Work out the finished part from the listing and answer in its coordinate system (mm). A direction names the side the tool comes from. Coordinates: 2 decimals unless noted, no trailing zeros. Order: outer loops, then holes, each group sorted by start corner. A loop starts at its lowest first (then second) coordinate and runs counter-clockwise, first axis right, second up. Notation, with made-up numbers: M -18.5,76.5 L -7.5,76.5 A6 ccw -7.5,81.5 Z; hole C 41,13 d10. An arc over 180 degrees is marked long. Use a Markdown table: item, result. Add a question column.
from build123d import *

# Parameters (mm, degrees)
SKETCH1_W           = 25
SKETCH1_H           = 25
BOSS_EXTRUDE1_DEPTH = 25
SHELL1_T            = 2.5
SKETCH2_W           = 12
SKETCH2_H           = 12
CUT_EXTRUDE1_DEPTH  = 15
SKETCH3_R           = 1.75
CUT_EXTRUDE2_DEPTH  = 15
SKETCH4_R           = 2.5
CUT_EXTRUDE6_DEPTH  = 15
SKETCH4_3_R         = 2.5
CUT_EXTRUDE7_DEPTH  = 15
SKETCH5_R           = 2.5
CUT_EXTRUDE8_DEPTH  = 15
SKETCH5_4_R         = 2.5
CUT_EXTRUDE9_DEPTH  = 15
SKETCH5_5_R         = 2.5
CUT_EXTRUDE10_DEPTH = 15
SKETCH7_R           = 2.5
CUT_EXTRUDE11_DEPTH = 15
SKETCH8_R           = 2.5
CUT_EXTRUDE12_DEPTH = 10


with BuildPart() as part:
    # Sketch1 → Boss-Extrude1 (new body)
    with BuildSketch(Plane(origin=(0, 0, 0), x_dir=(1, 0, 0), z_dir=(0, 1, 0))):
        Rectangle(SKETCH1_W, SKETCH1_H)
    extrude(amount=BOSS_EXTRUDE1_DEPTH)

    # Shell1 (no face opened: a closed hollow body)
    add(offset(amount=-SHELL1_T, mode=Mode.PRIVATE), mode=Mode.SUBTRACT)

    # Sketch2 → Cut-Extrude1 (cut)
    with BuildSketch(Plane(origin=(0, 25, 0), x_dir=(1, 0, 0), z_dir=(0, 1, 0))):
        Rectangle(SKETCH2_W, SKETCH2_H)
    extrude(amount=-CUT_EXTRUDE1_DEPTH, mode=Mode.SUBTRACT)

    # Sketch3 → Cut-Extrude2 (cut)
    with BuildSketch(Plane.XZ):
        with Locations((-5, 8.25)):
            Circle(SKETCH3_R)
        with Locations((-5, 0)):
            Circle(SKETCH3_R)
        with Locations((-5, -8.25)):
            Circle(SKETCH3_R)
        with Locations((5, 8.25)):
            Circle(SKETCH3_R)
        with Locations((5, 0)):
            Circle(SKETCH3_R)
        with Locations((5, -8.25)):
            Circle(SKETCH3_R)
    extrude(amount=-CUT_EXTRUDE2_DEPTH, mode=Mode.SUBTRACT)

    # Sketch4 → Cut-Extrude6 (cut)
    with BuildSketch(Plane(origin=(12.5, 0, 0), x_dir=(0, 0, -1), z_dir=(1, 0, 0))):
        with Locations((-7, 19.5)):
            Circle(SKETCH4_R)
    extrude(amount=-CUT_EXTRUDE6_DEPTH, mode=Mode.SUBTRACT)

    # Sketch4<3> → Cut-Extrude7 (cut)
    with BuildSketch(Plane(origin=(12.5, 0, 0), x_dir=(0, 0, -1), z_dir=(1, 0, 0))):
        with Locations((0, 12.5)):
            Circle(SKETCH4_3_R)
        with Locations((7, 5.5)):
            Circle(SKETCH4_3_R)
    extrude(amount=-CUT_EXTRUDE7_DEPTH, mode=Mode.SUBTRACT)

    # Sketch5 → Cut-Extrude8 (cut)
    with BuildSketch(Plane.ZY.offset(12.5)):
        with Locations((-6, 18.5)):
            Circle(SKETCH5_R)
    extrude(amount=-CUT_EXTRUDE8_DEPTH, mode=Mode.SUBTRACT)

    # Sketch5<4> → Cut-Extrude9 (cut)
    with BuildSketch(Plane.ZY.offset(12.5)):
        with Locations((6, 18.5)):
            Circle(SKETCH5_4_R)
    extrude(amount=-CUT_EXTRUDE9_DEPTH, mode=Mode.SUBTRACT)

    # Sketch5<5> → Cut-Extrude10 (cut)
    with BuildSketch(Plane.ZY.offset(12.5)):
        with Locations((6, 6.5)):
            Circle(SKETCH5_5_R)
        with Locations((-6, 6.5)):
            Circle(SKETCH5_5_R)
    extrude(amount=-CUT_EXTRUDE10_DEPTH, mode=Mode.SUBTRACT)

    # Sketch7 → Cut-Extrude11 (cut)
    with BuildSketch(Plane.XY.offset(12.5)):
        with Locations((-7.5, 20)):
            Circle(SKETCH7_R)
        with Locations((0, 12.5)):
            Circle(SKETCH7_R)
        with Locations((7.5, 20)):
            Circle(SKETCH7_R)
        with Locations((7.5, 5)):
            Circle(SKETCH7_R)
        with Locations((-7.5, 5)):
            Circle(SKETCH7_R)
    extrude(amount=-CUT_EXTRUDE11_DEPTH, mode=Mode.SUBTRACT)

    # Sketch8 → Cut-Extrude12 (cut)
    with BuildSketch(Plane(origin=(0, 0, -12.5), x_dir=(-1, 0, 0), z_dir=(0, 0, -1))):
        with Locations((0, 18.5)):
            Circle(SKETCH8_R)
        with Locations((0, 6.5)):
            Circle(SKETCH8_R)
    extrude(amount=-CUT_EXTRUDE12_DEPTH, mode=Mode.SUBTRACT)


solid = part.part
(1) Straight lines are drawn through the part: line 1 (Z direction, x = 5, y = 1.5); line 2 (X direction, y = 2.25, z = 8.25); line 3 (X direction, y = 5, z = 11.6). For each, find the intervals that lie inside material, in ascending order.
(2) A cutting plane is placed at D-D on y = 23.25. Write down the section's boundary in (x, z).
(3) A cutting plane is placed at A-A on z = 0. Write down the section's boundary in (x, y), plus the area to 3 significant figures.
(4) The mould has two halves that part along X. Classify faces 1 (the flat face through (9.5, 22, 10)), 2 (the flat face through (0, 24, 6)), 3 (the flat face through (-12.5, 12, 0)), 4 (the flat face through (-3, 12, 12.5)): pulls with the +X half, pulls with the -X half, needs draft (parallel to the pull), parting line crosses it, or undercut.
(5) A cutting plane is placed at C-C on y = 14.5. Write down the section's boundary in (x, z).
(6) Which of the six approach directions +Z, -Z, +X, -X, +Y, -Y give full straight-line access (tool end or side, diameter ignored) to faces 5 (the cylindrical face through (-11.268, 7.251, 8.385)), 6 (the flat face through (-9.5, 3.1, 10)), 7 (the cylindrical face through (9, 22, 11)), 8 (the cylindrical face through (0, 9, -11)), 9 (the cylindrical face through (-6.75, 1.23, 0.08))?
(7) A cutting plane is placed at B-B on x = 0. Write down the section's boundary in (y, z).
From the geometry:
| question | item | result |
|---|---|---|
| 1 | line 1 | z = -12.5 to -10, -6.5 to -1.75, 1.75 to 6.5, 10 to 12.5 |
| 1 | line 2 | x = -12.5 to -6.75, -3.25 to 3.25, 6.75 to 12.5 |
| 1 | line 3 | x = -12.5 to -10, -5 to 5, 10 to 12.5 |
| 2 | outline | M -12.5,-12.5 L 12.5,-12.5 L 12.5,12.5 L -12.5,12.5 Z; hole M -6,-6 L 6,-6 L 6,6 L -6,6 Z |
| 3 | outline | M -12.5,0 L -6.75,0 L -6.75,2.5 L -10,2.5 L -10,22.5 L -6,22.5 L -6,25 L -12.5,25 Z; M -3.25,0 L 3.25,0 L 3.25,2.5 L -3.25,2.5 Z; M 6,22.5 L 10,22.5 L 10,15 L 12.5,15 L 12.5,25 L 6,25 Z; M 6.75,0 L 12.5,0 L 12.5,10 L 10,10 L 10,2.5 L 6.75,2.5 Z |
| 3 | area | 165 mm2 |
| 4 | face 1 | undercut |
| 4 | face 2 | undercut |
| 4 | face 3 | pulls with the -X half |
| 4 | face 4 | needs draft |
| 5 | outline | M -12.5,-12.5 L 12.5,-12.5 L 12.5,-1.5 L 10,-1.5 L 10,-10 L -10,-10 L -10,10 L -1.5,10 L -1.5,12.5 L -12.5,12.5 Z; M 1.5,10 L 10,10 L 10,1.5 L 12.5,1.5 L 12.5,12.5 L 1.5,12.5 Z |
| 6 | face 5 | -X |
| 6 | face 6 | none |
| 6 | face 7 | +Z |
| 6 | face 8 | -Z |
| 6 | face 9 | -Y |
| 7 | outline | M 0,-12.5 L 4,-12.5 L 4,-10 L 2.5,-10 L 2.5,10 L 10,10 L 10,12.5 L 0,12.5 Z; M 9,-12.5 L 16,-12.5 L 16,-10 L 9,-10 Z; M 15,10 L 22.5,10 L 22.5,6 L 25,6 L 25,12.5 L 15,12.5 Z; M 21,-12.5 L 25,-12.5 L 25,-6 L 22.5,-6 L 22.5,-10 L 21,-10 Z |
